Work out the finished part from the listing and answer in its coordinate system (mm). Face numbers are marked on the shaded views. A direction names the side the tool comes from. Coordinates: 2 decimals unless noted, no trailing zeros. Order: outer loops, then holes, each group sorted by start corner. A loop starts at its lowest first (then second) coordinate and runs counter-clockwise, first axis right, second up. Notation, with made-up numbers: (59.25, 17) - (66.25, 17) arc R30 cw to (66.25, 50) - close; hole circle Ø1 at (-33, 4). An arc over 180 degrees is marked (long way). Use CSV: the item, a comma, the result in double quotes. Start each with the question number.
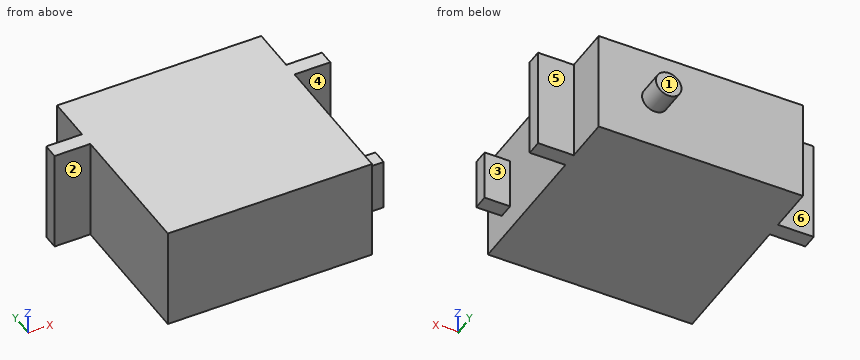
Autodesk Inventor part; units mm, degrees
ref_plane "Work Plane1" through (0, 0, 10) normal (0, 0, 1) x (1, 0, 0)
ref_plane "YZ Plane" through (0, 0, 0) normal (1, 0, 0) x (0, 1, 0)
ref_plane "XZ Plane" through (0, 0, 0) normal (0, 1, 0) x (-1, 0, 0)
sketch "Sketch1" plane through (0, 0, 0) normal (0, 0, 1) x (1, 0, 0)
  line L0 (-40, 0) -> (0, 0)
  line L1 (0, 0) -> (0, -7)
  line L2 (0, -7) -> (7, -7)
  line L3 (7, -7) -> (7, -10)
  line L4 (7, -10) -> (0, -10)
  line L5 (0, -10) -> (0, -30)
  line L6 (0, -38) -> (-40, -38)
  line L7 (-40, -38) -> (-40, -10)
  line L8 (-40, -10) -> (-47, -10)
  line L9 (-47, -10) -> (-47, -7)
  line L10 (-47, -7) -> (-40, -7)
  line L11 (-40, 0) -> (-40, -7)
  line L12 (0, -30) -> (5, -30)
  line L13 (5, -30) -> (5, -33)
  line L14 (5, -33) -> (0, -33)
  line L15 (0, -30) -> (0, -33) construction
  line L16 (0, -33) -> (0, -38)
  point P0 (7, -8.5)
  point P1 (-47, -8.5)
  point P2 (0, -24)
  dimension "d1" = 38
  dimension "d2" = 54
  dimension "d4" = 40
  dimension "d5" = 28
  dimension "d6" = 7
  dimension "d7" = 3
  dimension "d17" = 3
  dimension "d18" = 5
  dimension "d19" = 5
extrude "Extrusion1" add sketch "Sketch1" along normal blind 20
sketch "Sketch2" plane through (-40, 0, 0) normal (0, 1, 0) x (1, 0, 0)
  circle A0 centre (29, -10) radius 2.5
  line L0 (-7, 0) -> (-7, -20)
  line L1 (40, 0) -> (40, -20)
  line L2 (40, -10) -> (0, -10) construction
  line L3 (0, 0) -> (0, -20)
  line L4 (40, 0) -> (0, 0)
  line L5 (0, 0) -> (0, -20)
  line L6 (40, -20) -> (0, -20)
  line L7 (40, 0) -> (40, -20)
  dimension "d11" = 5
  dimension "d12" = 36
extrude "Extrusion2" add sketch "Sketch2" along normal blind 2 contours A0 | L1 L6 L3 L4
extrude "Extrusion3" add sketch "Sketch2" along normal blind 7 contours A0
sketch "Sketch3" plane through (0, -30, 0) normal (0, 1, 0) x (1, 0, 0)
  line L0 (5, 0) -> (0, 0)
  line L1 (0, 0) -> (0, -20)
  line L2 (5, -20) -> (0, -20)
  line L3 (5, 0) -> (5, -20)
  line L4 (0, 0) -> (0, -20)
  line L5 (5, 0) -> (5, -20)
  line L6 (0, -15) -> (5, -15)
  line L7 (5, -15) -> (5, -5)
  line L8 (5, -5) -> (0, -5)
  line L9 (0, -5) -> (0, -15)
  point P0 (0, -5)
  point P1 (5, -5)
  dimension "d20" = 5
  dimension "d21" = 5
extrude "Extrusion4" cut sketch "Sketch3" against normal through all contours L3 L8 L1 L0 | L3 L2 L1 L6
ref_plane "Work Plane1" through (0, 0, 10) normal (0, 0, 1) x (1, 0, 0)
properties part number "Servo_bigg_maketa"
1) The part is cut by section B-B on z = 2. Determine the outline of the cut face in (x, y).
2) For a pull along Y with two mould halves and no side action, classify the marked faces 1, 2 and 3 as +Y half, -Y half, draft (parallel to the pull), parting line (faces both ways), or undercut.
3) The part is cut by section D-D on z = 10. Determine the outline of the cut face in (x, y), plus the area to 3 significant figures.
4) Straight lines are drawn through the part: line 1 (Y direction, x = 0.5, z = 7); line 2 (X direction, y = -0.5, z = 18.25); line 3 (Y direction, x = -39, z = 9.25). For each, find the intervals that lie inside material, in ascending order. Write a range as [from, to].
5) Flat-ended cylindrical pins translate along their axes: P1, Ø5.5, axis at x = -45, z = 7.5, coming from the +Y side; P2, Ø4, axis at x = -3, y = -27.5, coming from the -Z side; P3, Ø3, axis at y = -4.5, z = 7, coming from the -X side; P4, Ø0.9, axis at y = -32, z = 8, coming from the +X side. Find the tip coordinate at first contact, or state that the pin passes through.
6) For the marked faces 4, 5 and 6, determine the directions among +Z, -Z, +X, -X, +Y, -Y from which every point of the face is accessible in a straight line to the end or side of a thin tool.
7) The part is cut by section C-C on y = 4.5. Determine the outline of the cut face in (x, z), plus the area to 3 significant figures.
8) The part is cut by section A-A on x = -11. Determine the outline of the cut face in (y, z).
Answer key:
1,outline,"(-47, -10) - (-40, -10) - (-40, -38) - (0, -38) - (0, -10) - (7, -10) - (7, -7) - (0, -7) - (0, 2) - (-40, 2) - (-40, -7) - (-47, -7) - close"
2,face 1,"+Y half"
2,face 2,"-Y half"
2,face 3,"undercut"
3,outline,"(-47, -10) - (-40, -10) - (-40, -38) - (0, -38) - (0, -33) - (5, -33) - (5, -30) - (0, -30) - (0, -10) - (7, -10) - (7, -7) - (0, -7) - (0, 2) - (-8.5, 2) - (-8.5, 7) - (-13.5, 7) - (-13.5, 2) - (-40, 2) - (-40, -7) - (-47, -7) - close"
3,area,"1,680 mm^2"
4,line 1,"[-33, -30], [-10, -7]"
4,line 2,"[-40, 0]"
4,line 3,"[-38, 2]"
5,P1,"y = -7"
5,P2,"z = 0"
5,P3,"x = -40"
5,P4,"x = 5"
6,face 4,"+Z, -Z, +X"
6,face 5,"+Z, -Z, +X, +Y"
6,face 6,"+Z, -Z, -X, +Y"
7,outline,"circle Ø5 at (-11, 10)"
7,area,"19.6 mm^2"
8,outline,"(-38, 0) - (2, 0) - (2, 7.5) - (7, 7.5) - (7, 12.5) - (2, 12.5) - (2, 20) - (-38, 20) - close"
